```python
from build123d import *

# Parameters (mm, degrees)
EXTRUDE_1_DEPTH = 150
EXTRUDE_3_DEPTH = 5
EXTRUDE_3_TAPER = 28
SHELL_9_T       = -2
FILLET_22_R     = 10


with BuildPart() as part:
    # 草圖1 → 填料-伸長1 (new body)
    with BuildSketch(Plane.XY):
        with BuildLine():
            Line((-30, 52), (30, 52))
            ThreePointArc((30, 52), (37.071067812, 49.071067812), (40, 42))
            Line((40, 42), (40, -42))
            ThreePointArc((40, -42), (37.071067812, -49.071067812), (30, -52))
            Line((30, -52), (-30, -52))
            ThreePointArc((-30, -52), (-37.071067812, -49.071067812), (-40, -42))
            Line((-40, -42), (-40, 42))
            ThreePointArc((-40, 42), (-37.071067812, 49.071067812), (-30, 52))
        make_face()
    extrude(amount=EXTRUDE_1_DEPTH)

    # 草圖3 → 填料-伸長3 (add)
    with BuildSketch(Plane.XY.offset(150)):
        with BuildLine():
            ThreePointArc((-30, 52), (-37.071067812, 49.071067812), (-40, 42))
            Line((-40, 42), (-40, -42))
            ThreePointArc((-40, -42), (-37.071067812, -49.071067812), (-30, -52))
            Line((-30, -52), (30, -52))
            ThreePointArc((30, -52), (37.071067812, -49.071067812), (40, -42))
            Line((40, -42), (40, 42))
            ThreePointArc((40, 42), (37.071067812, 49.071067812), (30, 52))
            Line((30, 52), (-30, 52))
        make_face()
    extrude(amount=EXTRUDE_3_DEPTH, taper=EXTRUDE_3_TAPER)

    # 薄殼9
    shell_9_openings = [part.faces().sort_by_distance(p)[0] for p in [
        (0, 0, 0),
    ]]
    offset(amount=SHELL_9_T, openings=shell_9_openings, kind=Kind.INTERSECTION)

    # 圓角22
    # the kernel refuses this fillet: 10 mm, written as the material it takes off along each edge
    with BuildSketch(Plane(origin=(-30, -42, 155), x_dir=(-1, 0, 0), z_dir=(0, 1, 0))) as fillet_22_piece_1:
        with BuildLine():
            CenterArc((1.339745962, -10), FILLET_22_R, 30, 60)
            Line((10, -5), (10.173205081, -4.9))
            ThreePointArc((10.173205081, -4.9), (8.847315939, -2.406105687), (7.51804236, 0.093894313))
            Line((7.51804236, 0.093894313), (7.341452842, 0.2))
            Line((7.341452842, 0.2), (1.339745962, 0.2))
            Line((1.339745962, 0.2), (1.339745962, 0))
        make_face()
    revolve(axis=Axis((-30, -42, 155), (0, 0, 1)), revolution_arc=90, mode=Mode.SUBTRACT)
    with BuildSketch(Plane(origin=(-37.341452842, 42, 155), x_dir=(1, 0, 0), z_dir=(0, -1, 0)), Plane(origin=(37.341452842, -42, 155), x_dir=(-1, 0, 0), z_dir=(0, 1, 0))) as fillet_22_piece_2:
        with BuildLine():
            CenterArc((6.00170688, -10), FILLET_22_R, 90, 60)
            Line((-2.658547158, -5), (-2.831752239, -4.9))
            ThreePointArc((-2.831752239, -4.9), (-1.505863098, -2.406105687), (-0.176589519, 0.093894313))
            Line((-0.176589519, 0.093894313), (0, 0.2))
            Line((0, 0.2), (6.00170688, 0.2))
            Line((6.00170688, 0.2), (6.00170688, 0))
        make_face()
    extrude(amount=84, mode=Mode.SUBTRACT)
    with BuildSketch(Plane(origin=(-30, 42, 155), x_dir=(0, 1, 0), z_dir=(1, 0, 0))) as fillet_22_piece_3:
        with BuildLine():
            CenterArc((1.339745962, -10), FILLET_22_R, 30, 60)
            Line((1.339745962, 0), (1.339745962, 0.2))
            Line((1.339745962, 0.2), (7.341452842, 0.2))
            Line((7.341452842, 0.2), (7.51804236, 0.093894313))
            ThreePointArc((7.51804236, 0.093894313), (8.847315939, -2.406105687), (10.173205081, -4.9))
            Line((10.173205081, -4.9), (10, -5))
        make_face()
    revolve(axis=Axis((-30, 42, 155), (0, 0, 1)), revolution_arc=90, mode=Mode.SUBTRACT)
    with BuildSketch(Plane(origin=(30, 49.341452842, 155), x_dir=(0, 0.46947156278588964, -0.8829475928589275), z_dir=(-1, 0, 0))) as fillet_22_piece_4:
        with BuildLine():
            CenterArc((6.01184522, 9.99390827), FILLET_22_R, 208, 60)
            Line((-2.817630708, 5.299192642), (-2.994220227, 5.20529833))
            Line((-2.994220227, 5.20529833), (-0.176589519, -0.093894313))
            Line((-0.176589519, -0.093894313), (0, -0.2))
            ThreePointArc((0, -0.2), (2.831425127, -0.2), (5.655870354, -0.199878165))
            Line((5.655870354, -0.199878165), (5.662850253, 0))
        make_face()
    extrude(amount=60, mode=Mode.SUBTRACT)
    with BuildSketch(Plane(origin=(30, 42, 155), x_dir=(1, 0, 0), z_dir=(0, -1, 0))) as fillet_22_piece_5:
        with BuildLine():
            CenterArc((1.339745962, -10), FILLET_22_R, 30, 60)
            Line((1.339745962, 0), (1.339745962, 0.2))
            Line((1.339745962, 0.2), (7.341452842, 0.2))
            Line((7.341452842, 0.2), (7.51804236, 0.093894313))
            ThreePointArc((7.51804236, 0.093894313), (8.847315939, -2.406105687), (10.173205081, -4.9))
            Line((10.173205081, -4.9), (10, -5))
        make_face()
    revolve(axis=Axis((30, 42, 155), (0, 0, 1)), revolution_arc=90, mode=Mode.SUBTRACT)
    with BuildSketch(Plane(origin=(30, -42, 155), x_dir=(0, -1, 0), z_dir=(-1, 0, 0))) as fillet_22_piece_6:
        with BuildLine():
            CenterArc((1.339745962, -10), FILLET_22_R, 30, 60)
            Line((10, -5), (10.173205081, -4.9))
            ThreePointArc((10.173205081, -4.9), (8.847315939, -2.406105687), (7.51804236, 0.093894313))
            Line((7.51804236, 0.093894313), (7.341452842, 0.2))
            Line((7.341452842, 0.2), (1.339745962, 0.2))
            Line((1.339745962, 0.2), (1.339745962, 0))
        make_face()
    revolve(axis=Axis((30, -42, 155), (0, 0, 1)), revolution_arc=90, mode=Mode.SUBTRACT)
    with BuildSketch(Plane(origin=(-30, -49.341452842, 155), x_dir=(0, 1, 0), z_dir=(1, 0, 0))) as fillet_22_piece_7:
        with BuildLine():
            CenterArc((6.00170688, -10), FILLET_22_R, 90, 60)
            Line((-2.658547158, -5), (-2.831752239, -4.9))
            ThreePointArc((-2.831752239, -4.9), (-1.505863098, -2.406105687), (-0.176589519, 0.093894313))
            Line((-0.176589519, 0.093894313), (0, 0.2))
            Line((0, 0.2), (6.00170688, 0.2))
            Line((6.00170688, 0.2), (6.00170688, 0))
        make_face()
    extrude(amount=60, mode=Mode.SUBTRACT)


solid = part.part
```
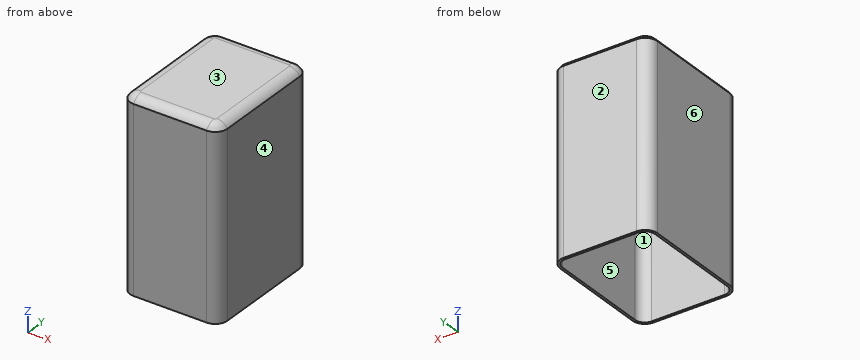
Input: part model. Units: mm. Frame: model coordinates. Face numbers are marked on the shaded views. A direction names the side the tool comes from. Coordinates: 2 decimals unless noted, no trailing zeros. Write each loop counter-clockwise with the first axis right and the second up, starting at its lowest first coordinate (ties: lowest second). Pieces come first, ordered by that corner, then holes.
1) Mould query, pull axis X, two halves, no side actions, for the marked faces 3, 4, 5 and 6. Classes: pulls with the +X half, pulls with the -X half, needs draft (parallel to the pull), parting line crosses it, or undercut.
2) Material intervals for line 1 along Y through (x, z) = (-3, 94); line 2 along X through (y, z) = (29, 11); line 3 along Z through (x, y) = (5.5, 10), sorted ascending.
3) Pin query (flat end, axial travel): pin 1 Ø6 at (x, y) = (-27.5, -2) entering from -Z. Return the tip coordinate at first contact, or that it passes through.
4) Set-up query: the marked faces 1 and 2. Return all of +Z, -Z, +X, -X, +Y, -Y with unobstructed straight access to the full face (end or side cutting, diameter ignored); none if empty.
5) Section A-A on z = 129. Output: boundary loops of the cut face in (x, y), and give its area (3 significant figures).
6) Section B-B on x = 15. Output: boundary loops of the cut face in (y, z), and give its area (3 significant figures).
7) Section C-C on y = -3. Output: boundary loops of the cut face in (x, z), and give its area (3 significant figures).
Check result:
1. face 3: needs draft
1. face 4: pulls with the +X half
1. face 5: undercut
1. face 6: pulls with the -X half
2. line 1: y = -52 to -50, 50 to 52
2. line 2: x = -40 to -38, 38 to 40
2. line 3: z = 153 to 155
3. pin 1: stops at z = 153
4. face 1: -Z
4. face 2: +Z, -Z, +X, -X, +Y
5. outline: (-40, -42) arc R10 ccw to (-30, -52) - (30, -52) arc R10 ccw to (40, -42) - (40, 42) arc R10 ccw to (30, 52) - (-30, 52) arc R10 ccw to (-40, 42) - close; hole (-38, -42) arc R8 ccw to (-30, -50) - (30, -50) arc R8 ccw to (38, -42) - (38, 42) arc R8 ccw to (30, 50) - (-30, 50) arc R8 ccw to (-38, 42) - close
5. area: 689 mm2
6. outline: (-52, 0) - (-50, 0) - (-50, 149.5) - (-48.14, 153) - (48.14, 153) - (50, 149.5) - (50, 0) - (52, 0) - (52, 150) arc R10 ccw to (43.34, 155) - (-43.34, 155) arc R10 ccw to (-52, 150) - close
6. area: 801 mm2
7. outline: (-40, 0) - (-38, 0) - (-38, 149.5) - (-36.14, 153) - (36.14, 153) - (38, 149.5) - (38, 0) - (40, 0) - (40, 150) arc R10 ccw to (31.34, 155) - (-31.34, 155) arc R10 ccw to (-40, 150) - close
7. area: 753 mm2
